The model under review builds one solid part; all positions refer to its coordinate system, in mm. A direction names the side the tool comes from. Coordinates: 2 decimals unless noted, no trailing zeros. Write each loop counter-clockwise with the first axis right and the second up, starting at its lowest first coordinate (ties: lowest second). Pieces come first, ordered by that corner, then holes.
```python
from build123d import *

# Parameters (mm, degrees)
F0_W     = 6.35
F0_H     = 12.7
F1_DEPTH = 1.5875


with BuildPart() as f1:
    # F0 (on Right) → F1 (new body, symmetric)
    with BuildSketch(Plane.YZ):
        Polygon((-1.5875, 18.950391), (-3.175, 6.35), (3.175, 6.35), (4.7625, 18.950391), (4.7625, 31.650391), align=None)
        Rectangle(F0_W, F0_H)
    extrude(amount=F1_DEPTH, both=True)


solid = f1.part
```
Item 1: Take a section at C-C, the plane y = -1. Write out the cut boundary in (x, z).
Solved:
outline: (-1.59, -6.35) - (1.59, -6.35) - (1.59, 20.13) - (-1.59, 20.13) - close
Item 2: Machinability: for faces 1 (the face through (0.022, 1.632, 25.389)), 2 (the face through (0, 3.175, 0)), which of the approach directions +Z, -Z, +X, -X, +Y, -Y give a long, thin tool a straight path to every point of the face, cutting with its end or side? Answer none if there is none.
Solved:
face 1: +Z, +X, -X, -Y
face 2: -Z, +X, -X, +Y
Item 3: Take a section at B-B, the plane z = 28.5. Write out the cut boundary in (x, y), plus the area to 3 significant figures.
Solved:
outline: (-1.59, 3.19) - (1.59, 3.19) - (1.59, 4.76) - (-1.59, 4.76) - close
area: 5.00 mm2
Item 4: To check wall thickness, follow line 1 along Y through (x, z) = (-0.7, 3.5) (3 decimals); line 2 along Z through (x, y) = (0.85, 1.25); line 3 along Y through (x, z) = (1.4, 8). State the ranges of each line that lie inside material, in increasing order.
Solved:
line 1: y = -3.175 to 3.175
line 2: z = -6.35 to 24.63
line 3: y = -2.97 to 3.38
Item 5: For pin 1 (1 mm diameter, centred on x = 1, y = 0, fed in from +Z); pin 2 (1.6 mm diameter, centred on x = -0.5, z = 0.5, fed in from +Y) (3 decimals), all flat-tipped, find the tip position at first contact; note any pin that passes through.
Solved:
pin 1: stops at z = 23.13
pin 2: stops at y = 3.175
